from build123d import *

# Parameters (mm, degrees)
F1_DEPTH = 20
F3_DEPTH = 20


with BuildPart() as f1:
    # F0 (on Front) → F1 (new body)
    with BuildSketch(Plane.XZ):
        Polygon((0, 40), (0, 0), (50, 0), align=None)
    extrude(amount=F1_DEPTH)

    # F2 (on face) → F3 (join)
    with BuildSketch(Plane.XZ.offset(20)):
        Polygon((31.8181818182, 14.5454545455), (10, 0), (40, 0), (40, 8), align=None)
        Polygon((40, 20), (31.8181818182, 14.5454545455), (40, 8), align=None)
    extrude(amount=F3_DEPTH)


solid = f1.part
Geometry check sheet. Reference: the model listing, model coordinates, mm. A direction names the side the tool comes from. Coordinates: 2 decimals unless noted, no trailing zeros. Order: outer loops, then holes, each group sorted by start corner. A loop starts at its lowest first (then second) coordinate and runs counter-clockwise, first axis right, second up. Notation, with made-up numbers: (76, 73) - (119, 73) arc R16 ccw to (119, 103) - close; hole circle Ø10 at (19.25, 32.5). An arc over 180 degrees is marked (long way). One line per item, written item: value.
(1) Sectioned sample at C-C (y = -17.5). Enter the section's corners in (x, z), and give its area (3 significant figures).
Data:
outline: (0, 0) - (50, 0) - (0, 40) - close
area: 1,000 mm^2
(2) Thickness scan on probe 1 along Y at (x, z) = (43, 2.5); probe 2 along X at (y, z) = (-32, 5.5); probe 3 along Z at (x, y) = (43, -6). Record the ranges inside material, lowest first. Write a range as from..to.
Data:
probe 1: y = -20..0
probe 2: x = 18.25..40
probe 3: z = 0..5.6
(3) Sectioned sample at D-D (z = 3.5). Enter the section's corners in (x, y) (3 decimals), and give its area (3 significant figures).
Data:
outline: (0, -20) - (15.25, -20) - (15.25, -40) - (40, -40) - (40, -20) - (45.625, -20) - (45.625, 0) - (0, 0) - close
area: 1,410 mm^2
(4) Depth check by flat-ended pin: pin 1 Ø2 at (x, y) = (41, -20) entering from -Z; pin 2 Ø6 at (x, y) = (16.5, -4.5) entering from +Z; pin 3 Ø6.5 at (x, z) = (45.5, 2) entering from -Y; pin 4 Ø4 at (x, y) = (20.5, -31.5) entering from +Z. Enter the tip coordinate at first touch or a pass-through.
Data:
pin 1: stops at z = 0
pin 2: stops at z = 29.2
pin 3: stops at y = -20
pin 4: stops at z = 8.33
(5) Access from +Z, -Z, +X, -X, +Y, -Y to the whole of each face (thin tool, end or side, straight path). Record for faces 1 (the face through (12, -20, 16)), 2 (the face through (14, 0, 11)), 3 (the face through (0, -10, 20)), 4 (the face through (40, -30, 10)), 5 (the face through (38, -20, 14)).
Data:
face 1: +Z, -X, -Y
face 2: +Z, -Z, +X, -X, +Y
face 3: +Z, -Z, -X, +Y, -Y
face 4: +Z, -Z, +X, -Y
face 5: +Z, +X, +Y
(6) Sectioned sample at B-B (x = 34). Enter the section's corners in (y, z).
Data:
outline: (-40, 0) - (0, 0) - (0, 12.8) - (-20, 12.8) - (-20, 16) - (-40, 16) - close
(7) Sectioned sample at A-A (z = 13.5). Enter the section's corners in (x, y) (3 decimals).
Data:
outline: (0, -20) - (30.25, -20) - (30.25, -40) - (40, -40) - (40, -20) - (33.125, -20) - (33.125, 0) - (0, 0) - close
